Here's how the part is built. I have some questions about the finished solid (model axes, mm). A direction names the side the tool comes from. Give positions to 0.01 mm unless a question says otherwise; leave off trailing zeros. Write each loop counter-clockwise with the first axis right and the second up, starting at its lowest first coordinate (ties: lowest second). Pieces come first, ordered by that corner, then holes. Notation, with made-up numbers: (49.5, 64.5) -> (88.5, 64.5) arc R17 ccw to (88.5, 78.5) -> close; hole circle Ø11 at (18, 11). An arc over 180 degrees is marked (long way). Answer as CSV lines item,"result". Start each with the question number.
Autodesk Inventor part; units mm, degrees
ref_plane "YZ Plane" through (0, 0, 0) normal (1, 0, 0) x (0, 1, 0)
ref_plane "XZ Plane" through (0, 0, 0) normal (0, 1, 0) x (-1, 0, 0)
ref_plane "XY Plane" through (0, 0, 0) normal (0, 0, 1) x (1, 0, 0)
sketch "Sketch2" plane through (0, 0, 0) normal (0, 0, 1) x (1, 0, 0)
  line L0 (5, 5) -> (70, 5)
  line L1 (70, 5) -> (70, 40)
  line L2 (70, 40) -> (5, 40)
  line L3 (5, 40) -> (5, 5)
  line L4 (15, 5) -> (20, 5)
  line L5 (20, 5) -> (20, 0)
  line L6 (20, 0) -> (15, 0)
  line L7 (15, 0) -> (15, 5)
  line L8 (30, 5) -> (30, 0)
  line L9 (30, 0) -> (25, 0)
  line L10 (25, 0) -> (25, 5)
  line L11 (40, 5) -> (40, 0)
  line L12 (40, 0) -> (35, 0)
  line L13 (35, 0) -> (35, 5)
  line L14 (50, 5) -> (50, 0)
  line L15 (50, 0) -> (45, 0)
  line L16 (45, 0) -> (45, 5)
  line L17 (60, 5) -> (60, 0)
  line L18 (60, 0) -> (55, 0)
  line L19 (55, 0) -> (55, 5)
  line L20 (70, 35) -> (75, 35)
  line L21 (75, 35) -> (75, 30)
  line L22 (75, 30) -> (70, 30)
  line L23 (70, 30) -> (70, 35)
  line L24 (75, 20) -> (70, 20)
  line L25 (70, 25) -> (75, 25)
  line L26 (75, 25) -> (75, 20)
  line L27 (75, 10) -> (70, 10)
  line L28 (70, 15) -> (75, 15)
  line L29 (75, 15) -> (75, 10)
  dimension "d122" = 10
  dimension "d129" = 65
  dimension "d132" = 10
extrude "Extrusion4" add sketch "Sketch2" along normal blind 5
properties part number "backside"
Item 1: I'm going to push flat-ended pins straight in: pin 1 (2.5 mm diameter, centred on x = 72.5, z = 2, fed in from -Y); pin 2 (3 mm diameter, centred on x = 62, z = 2, fed in from -Y); pin 3 (2 mm diameter, centred on x = 20, z = 3.5, fed in from -Y); pin 4 (2.5 mm diameter, centred on y = 1.5, z = 3, fed in from -X). Where does each tip first touch, or does it pass through?
Item 2: If I drill on line 1 (X direction, y = 4.5, z = 2.45); line 2 (X direction, y = 26, z = 1.1); line 3 (Y direction, x = 40.5, z = 3.35), over which ranges is the centre line in solid material (lowest first)? Write a range as [from, to].
Item 3: If we section it at B-B (x = 62.5): Please give me the cut outline in (y, z), and give its area (3 significant figures).
Item 4: We'd pull the mould along X, two halves only. Please class faces 6 (the face through (70, 27, 2)), 7 (the face through (22, 5, 2)), 8 (the face through (28, 0, 2)): released by +X, released by -X, zero draft, split by the parting line, or undercut.
Item 5: For faces 1 (the face through (15, 2, 2)), 2 (the face through (18, 0, 2)), 3 (the face through (50, 3, 2)), 4 (the face through (73, 30, 2)), 5 (the face through (73, 10, 2)), which set-ups out of +Z, -Z, +X, -X, +Y, -Y let a thin tool reach every point of the face, with its end or its side?
Item 6: If we section it at A-A (y = 3): Please give me the cut outline in (x, z).
Final values:
1,pin 1,"y = 10"
1,pin 2,"y = 5"
1,pin 3,"y = 0"
1,pin 4,"x = 15"
2,line 1,"[15, 20], [25, 30], [35, 40], [45, 50], [55, 60]"
2,line 2,"[5, 70]"
2,line 3,"[5, 40]"
3,outline,"(5, 0) -> (40, 0) -> (40, 5) -> (5, 5) -> close"
3,area,"175 mm2"
4,face 6,"released by +X"
4,face 7,"undercut"
4,face 8,"zero draft"
5,face 1,"+Z, -Z, -X, -Y"
5,face 2,"+Z, -Z, +X, -X, -Y"
5,face 3,"+Z, -Z, -Y"
5,face 4,"+Z, -Z, +X"
5,face 5,"+Z, -Z, +X, -Y"
6,outline,"(15, 0) -> (20, 0) -> (20, 5) -> (15, 5) -> close; (25, 0) -> (30, 0) -> (30, 5) -> (25, 5) -> close; (35, 0) -> (40, 0) -> (40, 5) -> (35, 5) -> close; (45, 0) -> (50, 0) -> (50, 5) -> (45, 5) -> close; (55, 0) -> (60, 0) -> (60, 5) -> (55, 5) -> close"
